For this review, take the finished solid that the model builds, in its own axes (mm). Face numbers are marked on the shaded views. Give positions to 0.01 mm unless a question says otherwise; leave off trailing zeros. Loops run counter-clockwise (first coordinate to the right, second up) from the corner with the lowest first, then second, coordinate; pieces in that order, holes last. Notation, with made-up numbers: (57, 53.5) -> (71, 53.5) arc R20 cw to (71, 88.5) -> close; hole circle Ø10 at (-0.75, 55.25). An arc over 180 degrees is marked (long way). One line per question, with ' | ' between items. Start each with the question number.
(1) Consider section A-A (z = 4.8). Write out the cut boundary in (x, y), and give its area (3 significant figures).
(2) Consider section B-B (y = -3.5). Write out the cut boundary in (x, z), and give its area (3 significant figures).
(3) Wall thickness on probe 1 along Y at (x, z) = (-16, 5.25); probe 2 along X at (y, z) = (-1.5, 0.85); probe 3 along Y at (x, z) = (-5, 5.15): over which ranges is each line inside the solid? List them lowest first.
(4) Consider section D-D (y = 17). Write out the cut boundary in (x, z), and give its area (3 significant figures).
(5) Draft analysis for pull direction X (two halves, no side actions). For the marked faces 1, 2 and 3, state which applies: +X half, -X half, draft (parallel to the pull), parting line (faces both ways), or undercut.
(6) Insertion check: P1, Ø4, axis at x = -3.5, y = 2.5, coming from the -Z side; P2, Ø3, axis at x = -8, y = -10.5, coming from the +Z side. Each pin has a flat end and moves straight along its axis. Give the tip position at first contact, or say it passes through.
(7) Consider section C-C (x = 16.5). Write out the cut boundary in (y, z), and give its area (3 significant figures).
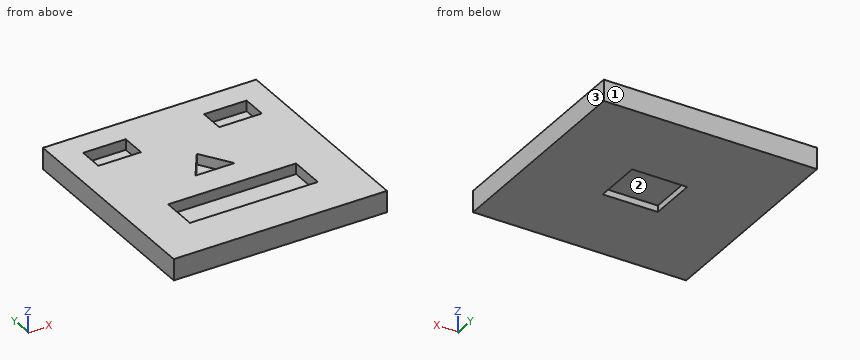
from build123d import *

# Parameters (mm, degrees)
F0_W     = 60
F0_H     = 60
F1_DEPTH = 6
F2_W     = 12
F2_H     = 7
F2_W_2   = 36
F2_H_2   = 10
F3_DEPTH = 3
F4_W     = 15.5
F4_H     = 13.5
F5_DEPTH = 1.8


with BuildPart() as f1:
    # F0 (on Top) → F1 (new body)
    with BuildSketch(Plane.XY):
        Rectangle(F0_W, F0_H)
    extrude(amount=F1_DEPTH)

    # F2 (on face) → F3 (cut)
    with BuildSketch(Plane.XY.offset(6)):
        with Locations((-17, 19.5)):
            Rectangle(F2_W, F2_H)
        with Locations((17, 19.5)):
            Rectangle(F2_W, F2_H)
        with Locations((0, -12.842694)):
            Rectangle(F2_W_2, F2_H_2)
        Polygon((5.5, 0), (0, 8.351647), (-5.5, 0), align=None)
    extrude(amount=-F3_DEPTH, mode=Mode.SUBTRACT)

    # F4 (on face) → F5 (cut)
    with BuildSketch(Plane(origin=(0, 0, 0), x_dir=(1, 0, 0), z_dir=(0, 0, -1))):
        Rectangle(F4_W, F4_H)
    extrude(amount=-F5_DEPTH, mode=Mode.SUBTRACT)


solid = f1.part
A:
1) outline: (-30, -30) -> (30, -30) -> (30, 30) -> (-30, 30) -> close; hole (-23, 16) -> (-11, 16) -> (-11, 23) -> (-23, 23) -> close; hole (-18, -17.84) -> (18, -17.84) -> (18, -7.84) -> (-18, -7.84) -> close; hole (-5.5, 0) -> (5.5, 0) -> (0, 8.35) -> close; hole (11, 16) -> (23, 16) -> (23, 23) -> (11, 23) -> close | area: 3,030 mm^2
2) outline: (-30, 0) -> (-7.75, 0) -> (-7.75, 1.8) -> (7.75, 1.8) -> (7.75, 0) -> (30, 0) -> (30, 6) -> (-30, 6) -> close | area: 332 mm^2
3) probe 1: y = -30 to -17.84, -7.84 to 16, 23 to 30 | probe 2: x = -30 to -7.75, 7.75 to 30 | probe 3: y = -30 to -17.84, -7.84 to 0, 0.76 to 30
4) outline: (-30, 0) -> (30, 0) -> (30, 6) -> (23, 6) -> (23, 3) -> (11, 3) -> (11, 6) -> (-11, 6) -> (-11, 3) -> (-23, 3) -> (-23, 6) -> (-30, 6) -> close | area: 288 mm^2
5) face 1: draft | face 2: undercut | face 3: +X half
6) P1: stops at z = 1.8 | P2: stops at z = 3
7) outline: (-30, 0) -> (30, 0) -> (30, 6) -> (23, 6) -> (23, 3) -> (16, 3) -> (16, 6) -> (-7.84, 6) -> (-7.84, 3) -> (-17.84, 3) -> (-17.84, 6) -> (-30, 6) -> close | area: 309 mm^2
